Can you work these out from the model? Positions are in its coordinate system, mm. A direction names the side the tool comes from. Coordinates: 2 decimals unless noted, no trailing zeros. Loops run counter-clockwise (first coordinate to the right, second up) from the corner with the lowest first, then second, coordinate; pieces in that order, holes last. Notation, with made-up numbers: (0, -13.75) - (43, -13.75) arc R16 ccw to (43, 13.25) - close; hole circle Ø7 at (31.25, 54). An arc over 180 degrees is marked (long way). Put each result on its own line as item: value. Start each with the question number.
from build123d import *

# Parameters (mm, degrees)
SKETCH1_R           = 76.2
SKETCH1_R_2         = 25.4
BOSS_EXTRUDE1_DEPTH = 7.366
SKETCH2_R           = 10.16
BOSS_EXTRUDE2_DEPTH = 5.334
SKETCH3_R           = 3.175
CUT_EXTRUDE1_DEPTH  = 109.014526597


with BuildPart() as part:
    # Sketch1 → Boss-Extrude1 (new body)
    with BuildSketch(Plane(origin=(0, 0, 0), x_dir=(1, 0, 0), z_dir=(0, 1, 0))):
        with Locations(Location((0, 0, 0), (0, 0, 270))):
            Circle(SKETCH1_R)
        with Locations(Location((0, 0, 0), (0, 0, 270))):
            Circle(SKETCH1_R_2, mode=Mode.SUBTRACT)
    extrude(amount=BOSS_EXTRUDE1_DEPTH)

    # Sketch2 → Boss-Extrude2 (add)
    with BuildSketch(Plane(origin=(0, 7.366, 0), x_dir=(1, 0, 0), z_dir=(0, 1, 0))):
        with Locations(Location((0, 50.8, 0), (0, 0, 270))):
            Circle(SKETCH2_R)
        with Locations(Location((-43.994090512, -25.4, 0), (0, 0, 270))):
            Circle(SKETCH2_R)
        with Locations(Location((43.994090512, -25.4, 0), (0, 0, 270))):
            Circle(SKETCH2_R)
    extrude(amount=BOSS_EXTRUDE2_DEPTH)

    # Sketch3 → Cut-Extrude1 (cut, through all)
    with BuildSketch(Plane(origin=(0, 7.366, 0), x_dir=(1, 0, 0), z_dir=(0, 1, 0))):
        with Locations(Location((-19.05, -64.77, 0), (0, 0, 270))):
            Circle(SKETCH3_R)
        with Locations(Location((19.05, -36.83, 0), (0, 0, 270))):
            Circle(SKETCH3_R)
        with Locations(Location((19.05, -64.77, 0), (0, 0, 90))):
            Circle(SKETCH3_R)
        with Locations(Location((-19.05, -36.83, 0), (0, 0, 90))):
            Circle(SKETCH3_R)
    extrude(amount=-CUT_EXTRUDE1_DEPTH, mode=Mode.SUBTRACT)


solid = part.part
Q1. On a 3-axis mill with a long thin cutter (end or side, diameter ignored), from which of +Z, -Z, +X, -X, +Y, -Y can I reach the whole of each face in a straight line? I mean faces 1 (the cylindrical face through (54.068, 9.996, 24.077)), 2 (the flat face through (44, 12.7, 25)). Say none if no direction works.
Q2. Will these pins go through, and if not, where does the flat tip stop? pin 1 (3 mm diameter, centred on y = 9, z = -56.5, fed in from +X); pin 2 (4 mm diameter, centred on x = -29.5, z = -43.5, fed in from +Y); pin 3 (5 mm diameter, centred on x = 19.05, z = 64.77, fed in from -Y); pin 4 (5 mm diameter, centred on y = 10, z = -44.5, fed in from -X).
Q3. I want a section at B-B on x = 0. List the corners of the cut face in (y, z) for me.
Q4. Please list where these lines run through material, in increasing order: line 1 along Z through (x, y) = (-1, 5.5); line 2 along X through (y, z) = (3, 36.5); line 3 along X through (y, z) = (2.75, 36.83) (3 decimals). Write a range as [from, to].
Q5. I want a section at A-A on z = 0. List the corners of the cut face in (x, y) for me, and give its area (3 significant figures).
Q6. I want a section at C-C on y = 1.75. List the corners of the cut face in (x, z) for me (3 decimals).
Q7. We'd pull the mould along Z, two halves only. Please class faces 3 (the flat face through (-33, 0, -1)), 4 (the cylindrical face through (-53.912, 9.996, 23.198)), 5 (the cylindrical face through (-15.95, 3.73, 37.52)): released by +Z, released by -Z, zero draft, split by the parting line, or undercut.
Q8. I want a section at D-D on x = 19.05. List the corners of the cut face in (y, z) for me (3 decimals).
Calculated:
1. face 1: +Y
1. face 2: +Z, -Z, +X, -X, +Y
2. pin 1: x = 9.25
2. pin 2: y = 7.37
2. pin 3: through
2. pin 4: x = -9.42
3. outline: (0, -76.2) - (7.37, -76.2) - (7.37, -60.96) - (12.7, -60.96) - (12.7, -40.64) - (7.37, -40.64) - (7.37, -25.4) - (0, -25.4) - close; (0, 25.4) - (7.37, 25.4) - (7.37, 76.2) - (0, 76.2) - close
4. line 1: [-76.19, -25.38], [25.38, 76.19]
4. line 2: [-66.89, -22.21], [-15.89, 15.89], [22.21, 66.89]
4. line 3: [-66.708, -22.225], [-15.875, 15.875], [22.225, 66.708]
5. outline: (-76.2, 0) - (-25.4, 0) - (-25.4, 7.37) - (-76.2, 7.37) - close; (25.4, 0) - (76.2, 0) - (76.2, 7.37) - (25.4, 7.37) - close
5. area: 748 mm2
6. outline: circle Ø152.4 at (0, 0); hole circle Ø50.8 at (0, 0); hole circle Ø6.35 at (-19.05, 36.83); hole circle Ø6.35 at (-19.05, 64.77); hole circle Ø6.35 at (19.05, 36.83); hole circle Ø6.35 at (19.05, 64.77)
7. face 3: zero draft
7. face 4: split by the parting line
7. face 5: undercut
8. outline: (0, -73.78) - (7.366, -73.78) - (7.366, -16.801) - (0, -16.801) - close; (0, 16.801) - (7.366, 16.801) - (7.366, 33.655) - (0, 33.655) - close; (0, 40.005) - (7.366, 40.005) - (7.366, 61.595) - (0, 61.595) - close; (0, 67.945) - (7.366, 67.945) - (7.366, 73.78) - (0, 73.78) - close
